Check sheet for the modelled part. Datum: model origin and axes. Units: mm. A direction names the side the tool comes from. Round coordinates to 2 decimals unless told otherwise and drop trailing zeros. Write each loop counter-clockwise with the first axis right and the second up, starting at its lowest first coordinate (ties: lowest second). Pieces come first, ordered by that corner, then holes. Notation, with made-up numbers: M -36.75,76 L 8.25,76 A26 cw 8.25,99 Z; hole C -0.75,45 d7. An arc over 180 degrees is marked long. Put each result on its own line as item: value.
```python
from build123d import *

# Parameters (mm, degrees)
F1_DEPTH = 76.2
F3_DEPTH = 25.4


with BuildPart() as f1:
    # F0 (on Top) → F1 (new body)
    with BuildSketch(Plane.XY):
        Polygon((-43.844193, 31.119447), (-43.844193, -32.380553), (-31.144193, -32.380553), (-31.144193, 18.419447), (19.655807, 18.419447), (19.655807, 31.119447), align=None)
    extrude(amount=F1_DEPTH)

    # F2 (on face) → F3 (cut)
    with BuildSketch(Plane.YZ.offset(-31.144193)):
        Polygon((-32.380553, 50.677463), (-32.380553, 0), (5.369338, 0), (5.369338, 25.450481), (-20.057857, 25.450481), (-20.057857, 37.863757), (-6.64351, 37.863757), (-6.64351, 50.677463), align=None)
    extrude(amount=-F3_DEPTH, mode=Mode.SUBTRACT)


solid = f1.part
```
1. Access from +Z, -Z, +X, -X, +Y, -Y to the whole of each face (thin tool, end or side, straight path). Record for faces 5 (the flat face through (-37, -20.058, 32)), 6 (the flat face through (-43.844, 7, 46)), 7 (the flat face through (-6, 18.419, 38)), 8 (the flat face through (-37, -13, 37.864)), 9 (the flat face through (19.656, 25, 38)).
Computed values:
face 5: -Z, +X, -X, -Y
face 6: +Z, -Z, -X, +Y, -Y
face 7: +Z, -Z, +X, -Y
face 8: +X, -X, -Y
face 9: +Z, -Z, +X, +Y, -Y
2. Cross-section at C-C (x = -4). Enter the section's corners in (y, z), then the cut area to 3 significant figures.
Computed values:
outline: M 18.42,0 L 31.12,0 L 31.12,76.2 L 18.42,76.2 Z
area: 968 mm2
3. Cross-section at D-D (y = -2). Enter the section's corners in (x, z), then the cut area to 3 significant figures.
Computed values:
outline: M -43.84,25.45 L -31.14,25.45 L -31.14,76.2 L -43.84,76.2 Z
area: 645 mm2
4. Scan lines: probe 1 along X at (y, z) = (15, 23); probe 2 along Y at (x, z) = (14, 15.5); probe 3 along Y at (x, z) = (-37, 26). Record each from-to range of solid material in increasing order.
Computed values:
probe 1: x = -43.84 to -31.14
probe 2: y = 18.42 to 31.12
probe 3: y = -20.06 to 31.12
5. Cross-section at A-A (y = -9.5). Enter the section's corners in (x, z).
Computed values:
outline: M -43.84,25.45 L -31.14,25.45 L -31.14,37.86 L -43.84,37.86 Z; M -43.84,50.68 L -31.14,50.68 L -31.14,76.2 L -43.84,76.2 Z
6. Cross-section at B-B (z = 26.5). Enter the section's corners in (x, y).
Computed values:
outline: M -43.84,-20.06 L -31.14,-20.06 L -31.14,18.42 L 19.66,18.42 L 19.66,31.12 L -43.84,31.12 Z
7. Release check for a two-part mould opening along Z. For faces 1 (the flat face through (-37, -19, 50.677)), 2 (the flat face through (-31.144, -2, 46)), 3 (the flat face through (-34, 14, 76.2)), 4 (the flat face through (-37, -6.644, 44)) record: +Z half, -Z half, draft (parallel to the pull), parting line (faces both ways), or undercut.
Computed values:
face 1: undercut
face 2: draft
face 3: +Z half
face 4: undercut
8. Depth check by flat-ended pin: pin 1 Ø10 at (x, z) = (-37.5, 43.5) entering from -Y; pin 2 Ø10 at (x, y) = (-36.5, -18.5) entering from -Z; pin 3 Ø5 at (y, z) = (9.5, 35.5) entering from +X. Enter the tip coordinate at first touch or a pass-through.
Computed values:
pin 1: stops at y = -6.64
pin 2: stops at z = 25.45
pin 3: stops at x = -31.14
